Verification items for this drawing (mm, ordinates from the low corner). A direction names the side the tool comes from. Round coordinates to 2 decimals unless told otherwise and drop trailing zeros. Write each loop counter-clockwise with the first axis right and the second up, starting at its lowest first coordinate (ties: lowest second). Pieces come first, ordered by that corner, then holes. Notation, with made-up numbers: (32, 39) -> (44, 39) arc R34 cw to (44, 71) -> close; hole circle Ø6 at (30, 0). An arc over 180 degrees is marked (long way). Put each result on its own line as item: value. Start each with the question number.
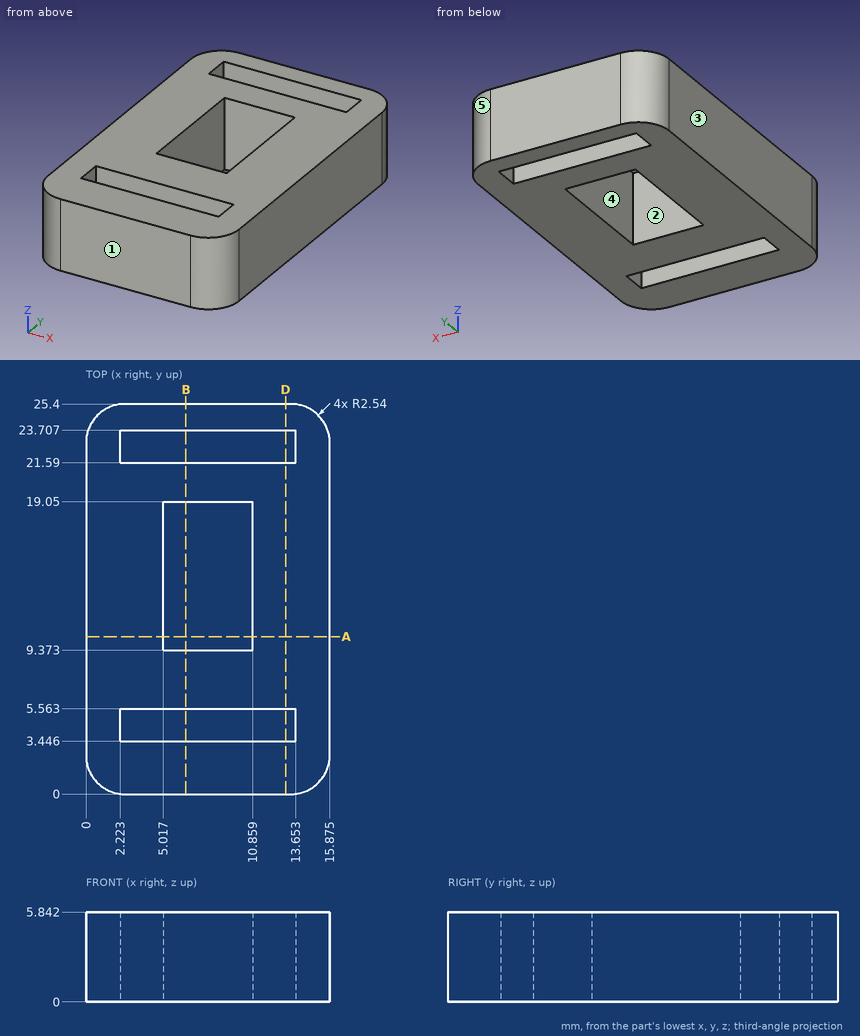
1. Section check A-A, the plane y = 10.25. Enter the section's corners in (x, z) (1 decimal).
2. Section check B-B, the plane x = 6.5. Give the number of separate pieces and of enclosed holes in the cut face.
3. Draft check along Y on the marked faces 1, 2 and 3. Enter one of: released by +Y, released by -Y, zero draft, split by the parting line, or undercut.
4. Material ranges on L1, parallel to Y at x = 4.25, z = 5.6 (1 decimal); L2, parallel to X at y = 4, z = 5.3 (1 decimal); L3, parallel to X at y = 13.5, z = 0.3 (1 decimal), recorded low to high. Write a range as [from, to].
5. Section check D-D, the plane x = 13. Enter the section's corners in (y, z) (1 decimal).
6. Access from +Z, -Z, +X, -X, +Y, -Y to the whole of each face (thin tool, end or side, straight path). Record for the marked faces 4 and 5.
Reply:
1. outline: (0, 0) -> (5, 0) -> (5, 5.8) -> (0, 5.8) -> close; (10.9, 0) -> (15.9, 0) -> (15.9, 5.8) -> (10.9, 5.8) -> close
2. separate pieces: 4
2. enclosed holes: 0
3. face 1: released by -Y
3. face 2: undercut
3. face 3: zero draft
4. L1: y = [0, 3.4], [5.6, 21.6], [23.7, 25.4]
4. L2: x = [0, 2.2], [13.7, 15.9]
4. L3: x = [0, 5], [10.9, 15.9]
5. outline: (0, 0) -> (3.4, 0) -> (3.4, 5.8) -> (0, 5.8) -> close; (5.6, 0) -> (21.6, 0) -> (21.6, 5.8) -> (5.6, 5.8) -> close; (23.7, 0) -> (25.4, 0) -> (25.4, 5.8) -> (23.7, 5.8) -> close
6. face 4: +Z, -Z
6. face 5: +Z, -Z, +X, +Y
